Here's how the part is built. I have some questions about the finished solid (model axes, mm). A direction names the side the tool comes from. Round coordinates to 2 decimals unless told otherwise and drop trailing zeros. Order: outer loops, then holes, each group sorted by start corner. A loop starts at its lowest first (then second) coordinate and runs counter-clockwise, first axis right, second up. Notation, with made-up numbers: (24, -24) -> (33, -24) arc R19 ccw to (33, 8) -> close; hole circle Ø9 at (44, 43). An arc over 180 degrees is marked (long way). Use a Markdown table: item, result. Add a question column.
Autodesk Inventor part; units mm, degrees
ref_plane "YZ Plane" through (0, 0, 0) normal (1, 0, 0) x (0, 1, 0)
ref_plane "XZ Plane" through (0, 0, 0) normal (0, 1, 0) x (-1, 0, 0)
ref_plane "XY Plane" through (0, 0, 0) normal (0, 0, 1) x (1, 0, 0)
ref_plane "Work Plane5" through (0, 3, 0) normal (0, 1, 0) x (1, 0, 0)
sketch "Sketch45" plane through (0, 3, 0) normal (0, 1, 0) x (1, 0, 0)
  line L0 (35, -20) -> (-3, -20)
  line L1 (-3, -20) -> (-3, 20)
  line L2 (-3, 20) -> (35, 20)
  line L3 (35, 20) -> (35, -20)
  point P0 (0, 0)
  dimension "d142" = 38
  dimension "d143" = 40
extrude "Extrusion34" add sketch "Sketch45" along normal blind 30
ref_plane "Work Plane2" through (0, 0, 0) normal (0, -1, 0) x (1, 0, 0)
sketch "Sketch47" plane through (0, 0, 0) normal (0, -1, 0) x (1, 0, 0)
  circle A0 centre (16, 0) radius 18
  point P0 (0, 0)
  dimension "d146" = 36
extrude "Extrusion35" cut sketch "Sketch47" against normal blind 30 draft -15
ref_plane "Work Plane1" through (0, 3, 0) normal (0, 1, 0) x (1, 0, 0)
sketch "Sketch74" plane through (0, 33, 0) normal (0, 1, 0) x (1, 0, 0)
  circle A0 centre (20, 0) radius 1.15
  point P0 (0, 0)
  dimension "d210" = 2.3
extrude "Extrusion51" cut sketch "Sketch74" against normal blind 10
sketch "Sketch77" plane through (0, 3, 0) normal (0, -1, 0) x (1, 0, 0)
  circle A0 centre (16, 0) radius 17.5
  point P0 (0, 0)
  dimension "d219" = 35
sketch "Sketch78" plane through (0, 3, 0) normal (0, -1, 0) x (1, 0, 0)
  line L0 (45, -30) -> (-13, -30)
  line L1 (-13, -30) -> (-13, 30)
  line L2 (-13, 30) -> (45, 30)
  line L3 (45, 30) -> (45, -30)
  line L4 (45, -30) -> (-13, 30) construction
  line L5 (-13, -30) -> (45, 30) construction
  point P0 (0, 0)
  point P1 (16, 0)
  dimension "d220" = 58
  dimension "d221" = 60
extrude "Extrusion53" add sketch "Sketch78" against normal blind 3
extrude "Extrusion54" cut sketch "Sketch77" against normal blind 3
sketch "Sketch81" plane through (0, 3, 0) normal (0, -1, 0) x (1, 0, 0)
  circle A0 centre (33.5, -25) radius 2.7
  line L0 (-13, -30) -> (45, -30)
  line L1 (45, -30) -> (45, 30)
  circle A1 centre (16, -25) radius 2.7
  circle A2 centre (-1.5, -25) radius 2.7
  circle A3 centre (-6.5, -8) radius 2.7
  circle A4 centre (-6.5, 8) radius 2.7
  circle A5 centre (-1.5, 25) radius 2.7
  circle A6 centre (16, 25) radius 2.7
  circle A7 centre (33.5, 25) radius 2.7
  point P0 (0, 0)
  dimension "mag_D" = 5.4
  dimension "d232" = 5
  dimension "d233" = 11.5
  dimension "d234" = 5.4
  dimension "d235" = 17.5
  dimension "d236" = 5.4
  dimension "d237" = 17.5
  dimension "d238" = 5.4
  dimension "d239" = 5
  dimension "d240" = 17
  dimension "d241" = 5.4
  dimension "d242" = 16
  dimension "d243" = 5.4
  dimension "d244" = 17
  dimension "d245" = 5.4
  dimension "d246" = 17.5
  dimension "d247" = 5.4
  dimension "d248" = 17.5
  dimension "d249" = 5
extrude "Extrusion56" cut sketch "Sketch81" against normal blind 30
sketch "Sketch83" plane through (0, 3, 0) normal (0, -1, 0) x (1, 0, 0)
  circle A0 centre (-6.5, -8) radius 2.7
  line L0 (-8.9107, -2) -> (-8.9107, 2)
  line L1 (-8.9107, 2) -> (-5.4466, 0)
  line L2 (-5.4466, 0) -> (-8.9107, -2)
  point P0 (0, 0)
  point P1 (-8.9107, -9.2159)
  point P2 (-7.756, 0)
  dimension "d253" = 4
extrude "Extrusion57" add sketch "Sketch83" along normal blind 4.5 contours L0 L1 L2
equation "\"d234\" = mag_D"
equation "\"d236\" = mag_D"
equation "\"d237\" = d235"
equation "\"d238\" = mag_D"
equation "\"d241\" = mag_D"
equation "\"d243\" = mag_D"
equation "\"d244\" = d240"
equation "\"d245\" = mag_D"
equation "\"d246\" = d235"
equation "\"d247\" = mag_D"
equation "\"d248\" = d235"
equation "\"d249\" = d239"
properties part number "liquid_port_v04"
(1) I'm going to push flat-ended pins straight in: P1, Ø6, axis at x = 33.5, z = 25, coming from the +Y side; P2, Ø4, axis at y = 28.5, z = 8.5, coming from the -X side; P3, Ø1.5, axis at x = 29, y = 14.5, coming from the -Z side. Where does each tip first touch, or does it pass through?
(2) I want a section at C-C on y = 13. List the corners of the cut face in (x, z) for me.
(3) I want a section at D-D on x = -6.5. List the corners of the cut face in (y, z) for me, and give its area (3 significant figures).
(4) Please list where these lines run through material, in increasing order: probe 1 along Z at (x, y) = (16, 5.2); probe 2 along Z at (x, y) = (-6.5, 3.7); probe 3 along Z at (x, y) = (24, 19.5). Write a range as from..to.
(5) I want a section at B-B on z = 25. List the corners of the cut face in (x, y) for me, and give its area (3 significant figures).
(6) On a 3-axis mill with a long thin cutter (end or side, diameter ignored), from which of +Z, -Z, +X, -X, +Y, -Y can I reach the whole of each face in a straight line? I mean faces 4 (the cylindrical face through (17.452, 4.479, 27.277)), 5 (the flat face through (-7.154, 0.781, -0.986)), 6 (the flat face through (16, 19, 20)). Say none if no direction works.
(7) If we mould it in two halves opening along Z, with no side actions, what happens to faces 1 (the flat face through (-7.203, 0.781, 1.014)), 2 (the flat face through (-3, 19, 0)), 3 (the cylindrical face through (17.452, 4.479, -22.723))? For each: pulls with the +Z half, pulls with the -Z half, needs draft (parallel to the pull), parting line crosses it, or undercut.
(8) I want a section at A-A on x = 16. List the corners of the cut face in (y, z) for me, and give its area (3 significant figures).
Output:
| question | item | result |
|---|---|---|
| 1 | P1 | y = 6 |
| 1 | P2 | x = -3 |
| 1 | P3 | z = -20 |
| 2 | outline | (-3, -20) -> (35, -20) -> (35, 20) -> (-3, 20) -> close; hole circle Ø29.03 at (16, 0) |
| 3 | outline | (-1.5, -0.61) -> (3, -0.61) -> (3, -5.3) -> (6, -5.3) -> (6, 5.3) -> (3, 5.3) -> (3, 0.61) -> (-1.5, 0.61) -> close; (3, -30) -> (6, -30) -> (6, -10.7) -> (3, -10.7) -> close; (3, 10.7) -> (6, 10.7) -> (6, 30) -> (3, 30) -> close |
| 3 | area | 153 mm² |
| 4 | probe 1 | -30..-27.7, -22.3..-17.5, 17.5..22.3, 27.7..30 |
| 4 | probe 2 | -30..-10.7, -5.3..5.3, 10.7..30 |
| 4 | probe 3 | -20..-9.96, 9.96..20 |
| 5 | outline | (-13, 3) -> (-4.2, 3) -> (-4.2, 6) -> (-13, 6) -> close; (1.2, 3) -> (13.3, 3) -> (13.3, 6) -> (1.2, 6) -> close; (18.7, 3) -> (30.8, 3) -> (30.8, 6) -> (18.7, 6) -> close; (36.2, 3) -> (45, 3) -> (45, 6) -> (36.2, 6) -> close |
| 5 | area | 125 mm² |
| 6 | face 4 | +Y, -Y |
| 6 | face 5 | -Z, +X, -Y |
| 6 | face 6 | +Z, +X, -X, +Y |
| 7 | face 1 | pulls with the +Z half |
| 7 | face 2 | needs draft |
| 7 | face 3 | undercut |
| 8 | outline | (3, -30) -> (6, -30) -> (6, -27.7) -> (3, -27.7) -> close; (3, -22.3) -> (6, -22.3) -> (6, -20) -> (33, -20) -> (33, 20) -> (6, 20) -> (6, 22.3) -> (3, 22.3) -> (3, 17.5) -> (6, 17.5) -> (6, 16.39) -> (30, 9.96) -> (30, -9.96) -> (6, -16.39) -> (6, -17.5) -> (3, -17.5) -> close; (3, 27.7) -> (6, 27.7) -> (6, 30) -> (3, 30) -> close |
| 8 | area | 490 mm² |
